```python
from build123d import *

# Parameters (mm, degrees)
MAIN_DEPTH                    = 3
MOTORCODERLEFTHOLE_DEPTH      = 4
SKETCH4_R                     = 1.5
BOTTOMLEFTHOLE_DEPTH          = 4
BOTTOMLEFTHOLELPATTERN_COUNT  = 5
BOTTOMLEFTHOLELPATTERN_PITCH  = 20
SKETCH5_R                     = 1.5
BOTTOMLEFTHOLE2_DEPTH         = 4
BOTTOMLEFTHOLE2LPATTERN_COUNT = 6
BOTTOMLEFTHOLE2LPATTERN_PITCH = 20
SKETCH6_R                     = 1.5
TOPLEFTHOLE_DEPTH             = 4
TOPLEFTHOLELPATTERN_COUNT     = 5
TOPLEFTHOLELPATTERN_PITCH     = 20
SKETCH7_R                     = 1.5
MOTORFIXHOLES_DEPTH           = 4
MOTORFIXHOLELPATTERN_COUNT    = 3
MOTORFIXHOLELPATTERN_PITCH    = 20
SKETCH8_R                     = 1.5
CODERHOLE_DEPTH               = 4
MIRROR1_COPY_1_SKETCH_R       = 1.5
MIRROR1_COPY_1_DEPTH          = 4
MIRROR1_COPY_2_SKETCH_R       = 1.5
MIRROR1_COPY_2_DEPTH          = 4
MIRROR1_COPY_3_SKETCH_R       = 1.5
MIRROR1_COPY_3_DEPTH          = 4
MIRROR1_COPY_4_SKETCH_R       = 1.5
MIRROR1_COPY_4_DEPTH          = 4
MIRROR1_COPY_5_SKETCH_R       = 1.5
MIRROR1_COPY_5_DEPTH          = 4
MIRROR1_COPY_6_SKETCH_R       = 1.5
MIRROR1_COPY_6_DEPTH          = 4
MIRROR1_COPY_7_SKETCH_R       = 1.5
MIRROR1_COPY_7_DEPTH          = 4
MIRROR1_COPY_8_SKETCH_R       = 1.5
MIRROR1_COPY_8_DEPTH          = 4
MIRROR1_COPY_9_SKETCH_R       = 1.5
MIRROR1_COPY_9_DEPTH          = 4
MIRROR1_COPY_10_SKETCH_R      = 1.5
MIRROR1_COPY_10_DEPTH         = 4
MIRROR1_COPY_11_SKETCH_R      = 1.5
MIRROR1_COPY_11_DEPTH         = 4
MIRROR1_COPY_12_SKETCH_R      = 1.5
MIRROR1_COPY_12_DEPTH         = 4
MIRROR1_COPY_13_SKETCH_R      = 1.5
MIRROR1_COPY_13_DEPTH         = 4
MIRROR1_COPY_14_SKETCH_R      = 1.5
MIRROR1_COPY_14_DEPTH         = 4
MIRROR1_COPY_15_SKETCH_R      = 1.5
MIRROR1_COPY_15_DEPTH         = 4
SKETCH3_R                     = 12
SKETCH3_R_2                   = 10
SKETCH3_R_3                   = 1.5
BIGHOLES_DEPTH                = 4


with BuildPart() as part:
    # Sketch1 → Main (new body)
    with BuildSketch(Plane.XY):
        Polygon((-60, 110), (-60, -110), (-40, -130), (40, -130), (40, -40), (20, -20), (20, 20), (40, 40), (40, 130), (-40, 130), align=None)
    extrude(amount=MAIN_DEPTH)

    # Sketch2 → MotorCoderLeftHole (cut, through all)
    with BuildSketch(Plane.XY.offset(3)):
        Polygon((-25, 100), (-25, 70), (25, 70), (25, 100), (15, 100), (15, 127), (-15, 127), (-15, 100), align=None)
    motorcoderlefthole = extrude(amount=-MOTORCODERLEFTHOLE_DEPTH, mode=Mode.SUBTRACT)

    # Sketch4 → BottomLeftHole (cut, through all)
    with BuildSketch(Plane.XY.offset(3)):
        with Locations((-55, 105)):
            Circle(SKETCH4_R)
    bottomlefthole = extrude(amount=-BOTTOMLEFTHOLE_DEPTH, mode=Mode.SUBTRACT)

    # BottomLeftHoleLPattern: BottomLeftHole ×5
    with Locations(*[(0, -i * BOTTOMLEFTHOLELPATTERN_PITCH, 0) for i in range(1, BOTTOMLEFTHOLELPATTERN_COUNT)]):
        add(bottomlefthole, mode=Mode.SUBTRACT)

    # Sketch5 → BottomLeftHole2 (cut, through all)
    with BuildSketch(Plane.XY.offset(3)):
        with Locations((-35, 125)):
            Circle(SKETCH5_R)
    bottomlefthole2 = extrude(amount=-BOTTOMLEFTHOLE2_DEPTH, mode=Mode.SUBTRACT)

    # BottomLeftHole2LPattern: BottomLeftHole2 ×6
    with Locations(*[(0, -i * BOTTOMLEFTHOLE2LPATTERN_PITCH, 0) for i in range(1, BOTTOMLEFTHOLE2LPATTERN_COUNT)]):
        add(bottomlefthole2, mode=Mode.SUBTRACT)

    # Sketch6 → TopLeftHole (cut, through all)
    with BuildSketch(Plane.XY.offset(3)):
        with Locations((35, 125)):
            Circle(SKETCH6_R)
    toplefthole = extrude(amount=-TOPLEFTHOLE_DEPTH, mode=Mode.SUBTRACT)

    # TopLeftHoleLPattern: TopLeftHole ×5
    with Locations(*[(0, -i * TOPLEFTHOLELPATTERN_PITCH, 0) for i in range(1, TOPLEFTHOLELPATTERN_COUNT)]):
        add(toplefthole, mode=Mode.SUBTRACT)

    # Sketch7 → MotorFixHoles (cut, through all)
    with BuildSketch(Plane.XY.offset(3)):
        with Locations((0, 65)):
            Circle(SKETCH7_R)
        with Locations((-10, 65)):
            Circle(SKETCH7_R)
        with Locations((10, 65)):
            Circle(SKETCH7_R)
    motorfixholes = extrude(amount=-MOTORFIXHOLES_DEPTH, mode=Mode.SUBTRACT)

    # MotorFixHoleLPattern: MotorFixHoles ×3
    with Locations(*[(0, -i * MOTORFIXHOLELPATTERN_PITCH, 0) for i in range(1, MOTORFIXHOLELPATTERN_COUNT)]):
        add(motorfixholes, mode=Mode.SUBTRACT)

    # Sketch8 → CoderHole (cut, through all)
    with BuildSketch(Plane.XY.offset(3)):
        with Locations((-45, 115)):
            Circle(SKETCH8_R)
        with Locations((-25, 115)):
            Circle(SKETCH8_R)
        with Locations((25, 115)):
            Circle(SKETCH8_R)
    coderhole = extrude(amount=-CODERHOLE_DEPTH, mode=Mode.SUBTRACT)

    # Mirror1: CoderHole, MotorCoderLeftHole, BottomLeftHole, BottomLeftHole2, TopLeftHole, MotorFixHoles across plane
    add(coderhole.mirror(Plane.ZX), mode=Mode.SUBTRACT)
    add(motorcoderlefthole.mirror(Plane.ZX), mode=Mode.SUBTRACT)
    add(bottomlefthole.mirror(Plane.ZX), mode=Mode.SUBTRACT)
    add(bottomlefthole2.mirror(Plane.ZX), mode=Mode.SUBTRACT)
    add(toplefthole.mirror(Plane.ZX), mode=Mode.SUBTRACT)
    add(motorfixholes.mirror(Plane.ZX), mode=Mode.SUBTRACT)

    # Mirror1 copy 1 sketch → Mirror1 copy 1 (cut, through all)
    with BuildSketch(Plane(origin=(0, 20, 3), x_dir=(1, 0, 0), z_dir=(0, 0, 1))):
        with Locations((35, -125)):
            Circle(MIRROR1_COPY_1_SKETCH_R)
    extrude(amount=-MIRROR1_COPY_1_DEPTH, mode=Mode.SUBTRACT)

    # Mirror1 copy 2 sketch → Mirror1 copy 2 (cut, through all)
    with BuildSketch(Plane(origin=(0, 40, 3), x_dir=(1, 0, 0), z_dir=(0, 0, 1))):
        with Locations((35, -125)):
            Circle(MIRROR1_COPY_2_SKETCH_R)
    extrude(amount=-MIRROR1_COPY_2_DEPTH, mode=Mode.SUBTRACT)

    # Mirror1 copy 3 sketch → Mirror1 copy 3 (cut, through all)
    with BuildSketch(Plane(origin=(0, 60, 3), x_dir=(1, 0, 0), z_dir=(0, 0, 1))):
        with Locations((35, -125)):
            Circle(MIRROR1_COPY_3_SKETCH_R)
    extrude(amount=-MIRROR1_COPY_3_DEPTH, mode=Mode.SUBTRACT)

    # Mirror1 copy 4 sketch → Mirror1 copy 4 (cut, through all)
    with BuildSketch(Plane(origin=(0, 80, 3), x_dir=(1, 0, 0), z_dir=(0, 0, 1))):
        with Locations((35, -125)):
            Circle(MIRROR1_COPY_4_SKETCH_R)
    extrude(amount=-MIRROR1_COPY_4_DEPTH, mode=Mode.SUBTRACT)

    # Mirror1 copy 5 sketch → Mirror1 copy 5 (cut, through all)
    with BuildSketch(Plane(origin=(0, 20, 3), x_dir=(1, 0, 0), z_dir=(0, 0, 1))):
        with Locations((-55, -105)):
            Circle(MIRROR1_COPY_5_SKETCH_R)
    extrude(amount=-MIRROR1_COPY_5_DEPTH, mode=Mode.SUBTRACT)

    # Mirror1 copy 6 sketch → Mirror1 copy 6 (cut, through all)
    with BuildSketch(Plane(origin=(0, 40, 3), x_dir=(1, 0, 0), z_dir=(0, 0, 1))):
        with Locations((-55, -105)):
            Circle(MIRROR1_COPY_6_SKETCH_R)
    extrude(amount=-MIRROR1_COPY_6_DEPTH, mode=Mode.SUBTRACT)

    # Mirror1 copy 7 sketch → Mirror1 copy 7 (cut, through all)
    with BuildSketch(Plane(origin=(0, 60, 3), x_dir=(1, 0, 0), z_dir=(0, 0, 1))):
        with Locations((-55, -105)):
            Circle(MIRROR1_COPY_7_SKETCH_R)
    extrude(amount=-MIRROR1_COPY_7_DEPTH, mode=Mode.SUBTRACT)

    # Mirror1 copy 8 sketch → Mirror1 copy 8 (cut, through all)
    with BuildSketch(Plane(origin=(0, 80, 3), x_dir=(1, 0, 0), z_dir=(0, 0, 1))):
        with Locations((-55, -105)):
            Circle(MIRROR1_COPY_8_SKETCH_R)
    extrude(amount=-MIRROR1_COPY_8_DEPTH, mode=Mode.SUBTRACT)

    # Mirror1 copy 9 sketch → Mirror1 copy 9 (cut, through all)
    with BuildSketch(Plane(origin=(0, 20, 3), x_dir=(1, 0, 0), z_dir=(0, 0, 1))):
        with Locations((-35, -125)):
            Circle(MIRROR1_COPY_9_SKETCH_R)
    extrude(amount=-MIRROR1_COPY_9_DEPTH, mode=Mode.SUBTRACT)

    # Mirror1 copy 10 sketch → Mirror1 copy 10 (cut, through all)
    with BuildSketch(Plane(origin=(0, 40, 3), x_dir=(1, 0, 0), z_dir=(0, 0, 1))):
        with Locations((-35, -125)):
            Circle(MIRROR1_COPY_10_SKETCH_R)
    extrude(amount=-MIRROR1_COPY_10_DEPTH, mode=Mode.SUBTRACT)

    # Mirror1 copy 11 sketch → Mirror1 copy 11 (cut, through all)
    with BuildSketch(Plane(origin=(0, 60, 3), x_dir=(1, 0, 0), z_dir=(0, 0, 1))):
        with Locations((-35, -125)):
            Circle(MIRROR1_COPY_11_SKETCH_R)
    extrude(amount=-MIRROR1_COPY_11_DEPTH, mode=Mode.SUBTRACT)

    # Mirror1 copy 12 sketch → Mirror1 copy 12 (cut, through all)
    with BuildSketch(Plane(origin=(0, 80, 3), x_dir=(1, 0, 0), z_dir=(0, 0, 1))):
        with Locations((-35, -125)):
            Circle(MIRROR1_COPY_12_SKETCH_R)
    extrude(amount=-MIRROR1_COPY_12_DEPTH, mode=Mode.SUBTRACT)

    # Mirror1 copy 13 sketch → Mirror1 copy 13 (cut, through all)
    with BuildSketch(Plane(origin=(0, 100, 3), x_dir=(1, 0, 0), z_dir=(0, 0, 1))):
        with Locations((-35, -125)):
            Circle(MIRROR1_COPY_13_SKETCH_R)
    extrude(amount=-MIRROR1_COPY_13_DEPTH, mode=Mode.SUBTRACT)

    # Mirror1 copy 14 sketch → Mirror1 copy 14 (cut, through all)
    with BuildSketch(Plane(origin=(0, 20, 3), x_dir=(1, 0, 0), z_dir=(0, 0, 1))):
        with Locations((0, -65)):
            Circle(MIRROR1_COPY_14_SKETCH_R)
        with Locations((-10, -65)):
            Circle(MIRROR1_COPY_14_SKETCH_R)
        with Locations((10, -65)):
            Circle(MIRROR1_COPY_14_SKETCH_R)
    extrude(amount=-MIRROR1_COPY_14_DEPTH, mode=Mode.SUBTRACT)

    # Mirror1 copy 15 sketch → Mirror1 copy 15 (cut, through all)
    with BuildSketch(Plane(origin=(0, 40, 3), x_dir=(1, 0, 0), z_dir=(0, 0, 1))):
        with Locations((0, -65)):
            Circle(MIRROR1_COPY_15_SKETCH_R)
        with Locations((-10, -65)):
            Circle(MIRROR1_COPY_15_SKETCH_R)
        with Locations((10, -65)):
            Circle(MIRROR1_COPY_15_SKETCH_R)
    extrude(amount=-MIRROR1_COPY_15_DEPTH, mode=Mode.SUBTRACT)

    # Sketch3 → BigHoles (cut, through all)
    with BuildSketch(Plane.XY.offset(3)):
        with Locations((-35, 0)):
            Circle(SKETCH3_R)
        with Locations((22.5, 55)):
            Circle(SKETCH3_R_2)
        with Locations((22.5, -55)):
            Circle(SKETCH3_R_2)
        Circle(SKETCH3_R_3)
        with Locations((-55, 0)):
            Circle(SKETCH3_R_3)
    extrude(amount=-BIGHOLES_DEPTH, mode=Mode.SUBTRACT)


solid = part.part
```
Build history of the part. All positions in model axes, mm. A direction names the side the tool comes from. Give positions to 0.01 mm unless a question says otherwise; leave off trailing zeros. Order: outer loops, then holes, each group sorted by start corner. A loop starts at its lowest first (then second) coordinate and runs counter-clockwise, first axis right, second up. Notation, with made-up numbers: M 70,54 L 128,54 A21 cw 128,82 Z; hole C 60,42 d2. An arc over 180 degrees is marked long. Write item = value, one per line. Start each with the question number.
(1) Slice it at C-C on y = -55. Write the cut outline in (x, z).
(2) Slice it at B-B on x = 30. Write the cut outline in (y, z), plus the area to 3 significant figures.
(3) Slice it at A-A on y = 76. Write the cut outline in (x, z), plus the area to 3 significant figures.
(4) Two-plate mould, pull along Y, no slides. Class faces 1 (the flat face through (-50, -120, 1)), 2 (the flat face through (-22, 2, 3)), 3 (the flat face through (30, -30, 1)): released by +Y, released by -Y, zero draft, split by the parting line, or undercut.
(5) Probe L1, parallel to Y at x = 2.5, z = 2.45; L2, parallel to Y at x = -22, z = 1.6; L3, parallel to X at y = 99, z = 2.2. List the from-to ranges inside material, lowest first. Write a range as [from, to].
(6) Which spindle directions (+Z, -Z, +X, -X, +Y, -Y) get a long thin tool onto all of the face, cutting with end or side? Do faces 4 (the flat face through (-50, 120, 1)), 5 (the flat face through (30, 30, 1)). Say none if no direction does.
(7) Pin check, flat tips, straight feed: pin 1 Ø1 at (x, z) = (-47, 0.5) entering from +Y; pin 2 Ø2.5 at (x, y) = (10, -65) entering from +Z; pin 3 Ø2 at (x, y) = (4.5, 6) entering from -Z. Stop position of each tip, or through.
Responses:
q1.outline = M -60,0 L 12.5,0 L 12.5,3 L -60,3 Z; M 32.5,0 L 40,0 L 40,3 L 32.5,3 Z
q2.outline = M -130,0 L -61.61,0 L -61.61,3 L -130,3 Z; M -48.39,0 L -30,0 L -30,3 L -48.39,3 Z; M 30,0 L 48.39,0 L 48.39,3 L 30,3 Z; M 61.61,0 L 130,0 L 130,3 L 61.61,3 Z
q2.area = 521 mm2
q3.outline = M -60,0 L -25,0 L -25,3 L -60,3 Z; M 25,0 L 40,0 L 40,3 L 25,3 Z
q3.area = 150 mm2
q4.face_1 = released by -Y
q4.face_2 = zero draft
q4.face_3 = undercut
q5.L1 = [-130, -127], [-70, 70], [127, 130]
q5.L2 = [-130, -100], [-70, 70], [100, 130]
q5.L3 = [-60, -25], [25, 40]
q6.face_4 = +Z, -Z, -X, +Y
q6.face_5 = +Z, -Z, +X
q7.pin_1 = 123.5
q7.pin_2 = through
q7.pin_3 = 0
